Here's the drawing with two shaded views (mm, measured from the low corner). I have some questions. Round coordinates to 2 decimals unless told otherwise and drop trailing zeros. Order: outer loops, then holes, each group sorted by start corner. A loop starts at its lowest first (then second) coordinate and runs counter-clockwise, first axis right, second up. Notation, with made-up numbers: (87.5, 18) - (144.5, 18) arc R15 cw to (144.5, 38) - close; hole circle Ø1 at (39, 15). An arc over 180 degrees is marked (long way). One line per item, written item: value.
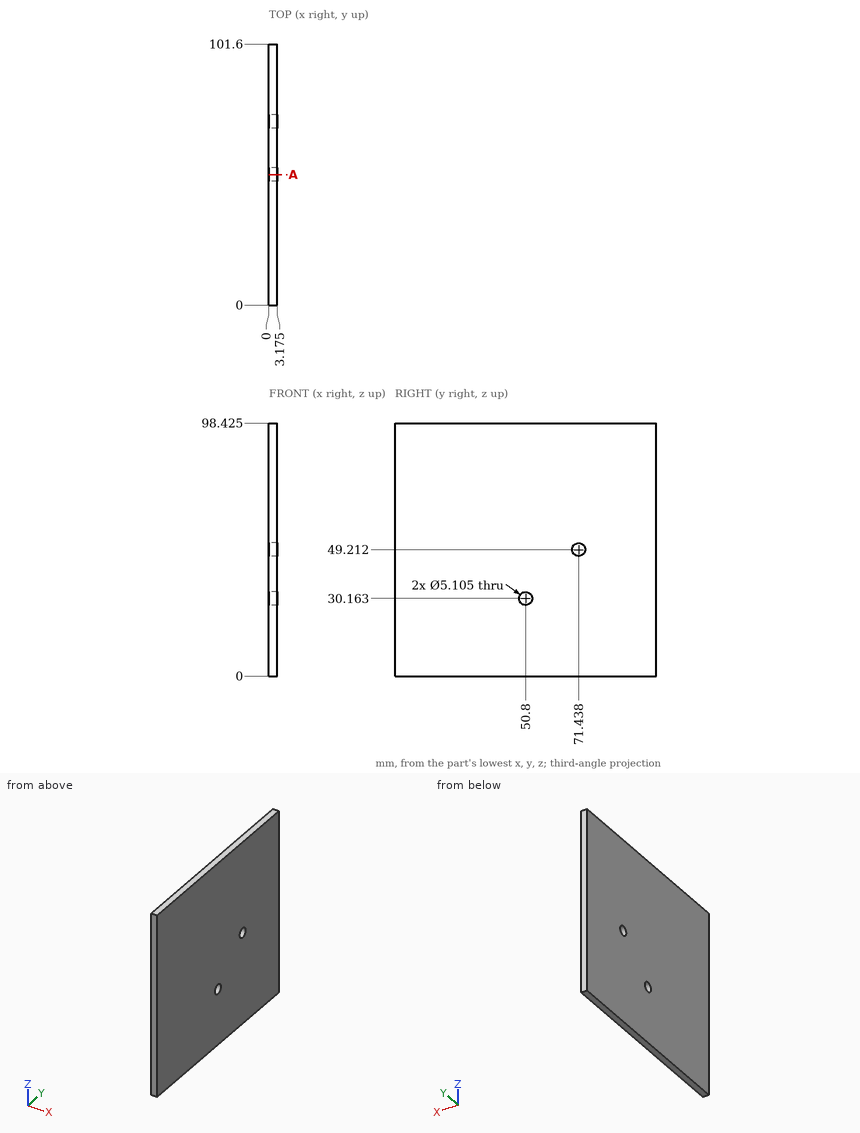
Q1. If I drill on line 1 along Z through (x, y) = (1.6, 50.8) (1 decimal); line 2 along Y through (x, z) = (1.7, 49); line 3 along Y through (x, z) = (1.25, 30.5), over which ranges is the centre line in solid material (lowest first)?
Results list:
line 1: 0 to 27.6, 32.7 to 98.4
line 2: 0 to 68.89, 73.98 to 101.6
line 3: 0 to 48.27, 53.33 to 101.6
Q2. If we section it at A-A, the plane y = 50.8: Please give me the cut outline in (x, z) (1 decimal).
Results list:
outline: (0, 0) - (3.2, 0) - (3.2, 27.6) - (0, 27.6) - close; (0, 32.7) - (3.2, 32.7) - (3.2, 98.4) - (0, 98.4) - close
Q3. Will this pin go through, and if not, where does the flat tip stop? pin 1 (3 mm diameter, centred on y = 71.44, z = 49.21, fed in from +X).
Results list:
pin 1: through
